The listing builds one solid part. Answer for the finished solid, in the listing's coordinates (mm). Give positions to 0.01 mm unless a question says otherwise; leave off trailing zeros. Write each loop counter-clockwise with the first axis right and the second up, starting at its lowest first coordinate (ties: lowest second). Pieces come first, ordered by that corner, then holes. Notation, with made-up numbers: M 22,9 L 63,9 A7 ccw 63,22 Z; hole C 6.25,42.5 d6. An arc over 180 degrees is marked long. Return JSON: item names as keys, results as strings.
Autodesk Fusion 360 part; units mm, degrees
sketch "brace" plane through (0, 0, 0) normal (0, 1, 0) x (1, 0, 0)
  line L0 (0, 0) -> (-83, 0)
  line L1 (-83, 0) -> (-83, 15)
  line L2 (-83, 15) -> (0, 15)
  line L3 (0, 15) -> (0, 0)
  dimension "d1" = 83
  dimension "d2" = 15
extrude "Extrude1" add sketch "brace" along normal blind 15
sketch "3mm hole" plane through (0, 0, 0) normal (1, 0, 0) x (0, 0, -1)
  line L0 (15, 0) -> (0, 0) construction
  line L1 (7.5, 0) -> (7.5, 7.5) construction
  circle A0 centre (7.5, 7.5) radius 1.425
  dimension "d5" = 7.5
  dimension "d6" = 2.85
sketch "side nut slot" plane through (0, 0, 0) normal (0, 0, 1) x (1, 0, 0)
  line L0 (0, 0) -> (-5.9, 0) construction
  line L1 (-5.9, 0) -> (-5.9, 4.65) construction
  line L2 (-5.9, 4.65) -> (-8.5, 4.65)
  line L3 (-8.5, 4.65) -> (-8.5, 10.35)
  line L4 (-8.5, 10.35) -> (-5.9, 10.35)
  line L5 (-5.9, 10.35) -> (-5.9, 4.65)
  line L6 (-83, 0) -> (-77.1, 0) construction
  line L7 (-77.1, 0) -> (-77.1, 4.65) construction
  line L8 (-77.1, 4.65) -> (-74.5, 4.65)
  line L9 (-74.5, 4.65) -> (-74.5, 10.35)
  line L10 (-74.5, 10.35) -> (-77.1, 10.35)
  line L11 (-77.1, 10.35) -> (-77.1, 4.65)
  point P0 (-83, 0)
  dimension "d7" = 5.9
  dimension "d8" = 4.65
  dimension "d9" = 2.6
  dimension "d10" = 5.7
  dimension "d11" = 5.9
  dimension "d12" = 4.65
  dimension "d13" = 2.6
  dimension "d14" = 5.7
extrude "Extrude2" cut sketch "side nut slot" against normal blind 12
extrude "Extrude3" cut sketch "3mm hole" against normal blind 10
extrude "Extrude4" cut sketch "3mm hole" along normal blind 10 from surface at -83
chamfer "Chamfer1" distance 0.5 angle 45 4 edges at (-77.1, 7.5, 0) (-75.8, 10.35, 0) (-74.5, 7.5, 0) (-75.8, 4.65, 0)
chamfer "Chamfer2" distance 0.5 angle 45 4 edges at (-7.2, 10.35, 0) (-5.9, 7.5, 0) (-7.2, 4.65, 0) (-8.5, 7.5, 0)
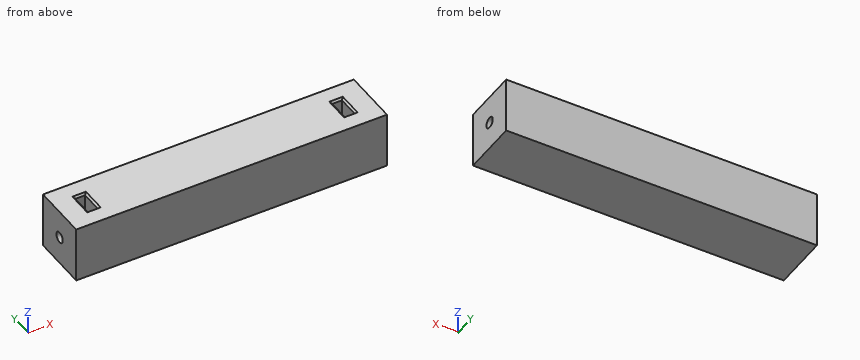
Item 1: Given pin 1 Ø6 at (x, y) = (-53.5, 7.5) entering from +Z; pin 2 Ø0.8 at (x, y) = (-76.5, 8) entering from +Z, each flat-ended and moving along its own axis, determine where each tip first touches the part or whether it passes through.
Geometry results:
{"pin 1": "stops at z = 0", "pin 2": "stops at z = -12"}
Item 2: A cutting plane is placed at A-A, the plane y = 7.5. Count the separate pieces of the cut face and the enclosed holes in it, plus the area to 3 significant figures.
Geometry results:
{"separate pieces": "3", "enclosed holes": "0", "area": "1,140 mm2"}
Item 3: A cutting plane is placed at C-C, the plane z = -7.5. Write down the section's boundary in (x, y) (3 decimals), plus the area to 3 significant figures.
Geometry results:
{"outline": "M -83,0 L 0,0 L 0,6.075 L -5.9,6.075 L -5.9,4.65 L -8.5,4.65 L -8.5,6.075 L -10,6.075 L -10,8.925 L -8.5,8.925 L -8.5,10.35 L -5.9,10.35 L -5.9,8.925 L 0,8.925 L 0,15 L -83,15 L -83,8.925 L -77.1,8.925 L -77.1,10.35 L -74.5,10.35 L -74.5,8.925 L -73,8.925 L -73,6.075 L -74.5,6.075 L -74.5,4.65 L -77.1,4.65 L -77.1,6.075 L -83,6.075 Z", "area": "1,170 mm2"}
Item 4: Find the intervals of material crossed by line 1 (X direction, y = 7.5, z = -1); line 2 (Y direction, x = -9.5, z = -7.5) (3 decimals), in increasing order.
Geometry results:
{"line 1": "x = -83 to -77.1, -74.5 to -8.5, -5.9 to 0", "line 2": "y = 0 to 6.075, 8.925 to 15"}
Item 5: A cutting plane is placed at B-B, the plane z = -2.25. Write down the section's boundary in (x, y).
Geometry results:
{"outline": "M -83,0 L 0,0 L 0,15 L -83,15 Z; hole M -77.1,4.65 L -74.5,4.65 L -74.5,10.35 L -77.1,10.35 Z; hole M -8.5,4.65 L -5.9,4.65 L -5.9,10.35 L -8.5,10.35 Z"}
